Print and shaded views of the part. All mm, measured from the part's lowest x, y and z. A direction names the side the tool comes from. Coordinates: 2 decimals unless noted, no trailing zeros. Order: outer loops, then holes, each group sorted by start corner. A loop starts at its lowest first (then second) coordinate and runs counter-clockwise, first axis right, second up. Notation, with made-up numbers: M 87.25,-11.75 L 100.25,-11.75 A17 ccw 100.25,-3.75 Z; hole C 26,-1.5 d5. An arc over 180 degrees is marked long. Use a Markdown table: item, result. Add a question column.
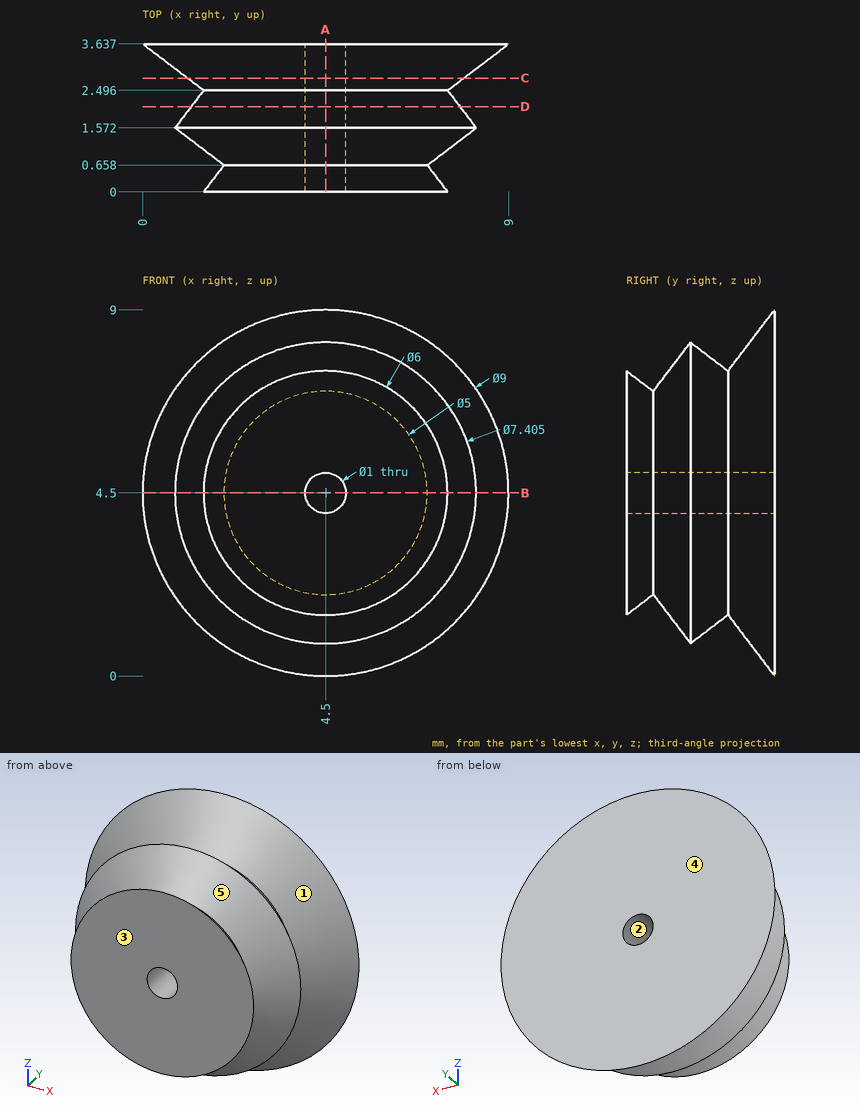
(1) Slice it at B-B on z = 4.5. Give the cut face in (x, y).
(2) Slice it at D-D on y = 2.1. Give the cut face in (x, z).
(3) Mould opens along X. For the marked faces 1, 2 and 3 say: released by +X, released by -X, zero draft, split by the parting line, or undercut.
(4) Drop a flat-ended pin along its axis: P1, Ø2, axis at y = 1, z = 3, coming from the +X side. Give the stop position or say it passes through.
(5) Slice it at C-C on y = 2.8. Give the cut face in (x, z).
(6) Slice it at A-A on x = 4.5. Give the cut face in (y, z).
(7) Drill centre lines: line 1 along Y through (x, z) = (7.75, 4.25) (1 decimal); line 2 along X through (y, z) = (2.85, 4.5) (1 decimal); line 3 along Y through (x, z) = (2, 5.5) (1 decimal). Where is each one in solid material? Low to high. Write a range as from..to.
(8) Which spindle directions (+Z, -Z, +X, -X, +Y, -Y) get a long thin tool onto all of the face, cutting with end or side? Do the marked faces 4 and 5. Say none if no direction does.
Solutions:
| question | item | result |
|---|---|---|
| 1 | outline | M 0,3.64 L 1.5,2.5 L 0.8,1.57 L 2,0.66 L 1.5,0 L 4,0 L 4,3.64 Z; M 5,0 L 7.5,0 L 7,0.66 L 8.2,1.57 L 7.5,2.5 L 9,3.64 L 5,3.64 Z |
| 2 | outline | C 4.5,4.5 d6.6; hole C 4.5,4.5 d1 |
| 3 | face 1 | split by the parting line |
| 3 | face 2 | undercut |
| 3 | face 3 | zero draft |
| 4 | P1 | x = 8.14 |
| 5 | outline | C 4.5,4.5 d6.8; hole C 4.5,4.5 d1 |
| 6 | outline | M 0,1.5 L 0.66,2 L 1.57,0.8 L 2.5,1.5 L 3.64,0 L 3.64,4 L 0,4 Z; M 0,5 L 3.64,5 L 3.64,9 L 2.5,7.5 L 1.57,8.2 L 0.66,7 L 0,7.5 Z |
| 7 | line 1 | 1.2..2.2, 2.7..3.6 |
| 7 | line 2 | 1..4, 5..8 |
| 7 | line 3 | 0..0.4, 0.8..3.6 |
| 8 | face 4 | +Z, -Z, +X, -X, +Y |
| 8 | face 5 | none |
